Autodesk Inventor part; units mm, degrees
ref_plane "Work Plane1" through (76.2, 0, -20.6375) normal (0, 0, -1) x (-1, 0, 0)
ref_plane "YZ Plane" through (0, 0, 0) normal (1, 0, 0) x (0, 1, 0)
ref_plane "XZ Plane" through (0, 0, 0) normal (0, 1, 0) x (-1, 0, 0)
sketch "Sketch1" plane through (0, 0, 0) normal (0, 1, 0) x (-1, 0, 0)
  line L0 (0, 0) -> (-76.2, 0)
  line L1 (-76.2, 0) -> (-76.2, -41.275)
  line L2 (-76.2, -41.275) -> (0, -41.275)
  line L3 (0, -41.275) -> (0, 0)
  line L4 (0, -39.6875) -> (-76.2, -39.6875)
  line L5 (0, -20.6375) -> (-76.2, -20.6375) construction
  dimension "d0" = 76.2
  dimension "d1" = 41.275
  dimension "d4" = 1.5875
extrude "Extrusion1" add sketch "Sketch1" against normal blind 1.5875
ref_plane "Work Plane1" through (76.2, 0, -20.6375) normal (0, 0, -1) x (-1, 0, 0)
extrude "Extrusion2" add sketch "Sketch1" along normal blind 4.1688 contours L3 L2 L1 L4
sketch "Sketch2" plane through (0, -1.5875, 0) normal (-1, 0, 0) x (0, 0, 1)
  line L0 (-41.275, 5.7563) -> (-39.6875, 5.7563) construction
  line L1 (-39.6875, 1.5875) -> (-39.6875, 5.7563) construction
  circle A0 centre (-39.6875, 4.9625) radius 0.7937
  dimension "d7" = 1.5875
extrude "Extrusion3" add sketch "Sketch2" against normal up to surface (76.2 mm away)
fillet "Fillet1" radius 1.5875 1 edges at (38.1, 4.1688, -41.275)
mirror "Mirror1" about plane through (76.2, 0, -20.6375) normal (0, 0, -1) of "Extrusion2", "Extrusion3", "Fillet1"
fillet "Fillet2" radius 1.5875 2 edges at (38.1, -1.5875, -41.275) (38.1, -1.5875, 0)
fillet "Fillet3" radius 0.7937 2 edges at (38.1, 0, -39.6875) (38.1, 0, -1.5875)
properties part number "Duct Cover"
The listing builds one solid part. Answer for the finished solid, in the listing's coordinates (mm). A direction names the side the tool comes from. Coordinates: 2 decimals unless noted, no trailing zeros. Loops run counter-clockwise (first coordinate to the right, second up) from the corner with the lowest first, then second, coordinate; pieces in that order, holes last. Notation, with made-up numbers: (89, -37.75) - (128, -37.75) arc R25 cw to (128, -2.75) - close; hole circle Ø1 at (-0.5, -2.5). An arc over 180 degrees is marked (long way). Write item = value, one per line.
1) Determine the mould class of faces 4 (the face through (39, 2, -1.588)), 5 (the face through (38.63, -1.11, -0.45)), 6 (the face through (76.2, -0.2, -20.7)) for opening direction Z: pulls with the +Z half, pulls with the -Z half, needs draft (parallel to the pull), parting line crosses it, or undercut.
Responses:
face_4 = undercut
face_5 = pulls with the +Z half
face_6 = needs draft
2) Which of the six approach directions +Z, -Z, +X, -X, +Y, -Y give full straight-line access (tool end or side, diameter ignored) to faces 1 (the face through (38, 1, 0)), 2 (the face through (39, 0, -20)), 3 (the face through (37.57, 3.39, -2.38))?
Responses:
face_1 = +Z, +X, -X, +Y, -Y
face_2 = +X, -X, +Y
face_3 = +X, -X
3) Find the intervals of material crossed by line 1 along Z through (x, y) = (33.5, 1.35) (1 decimal); line 2 along Y through (x, z) = (59.5, -20); line 3 along Z through (x, y) = (71.5, -0.15), in increasing order.
Responses:
line_1 = -41.3 to -39.7, -1.6 to 0
line_2 = -1.59 to 0
line_3 = -41.27 to -0.01
4) This flat-tipped pin is pushed along its axis until it touches: P1, Ø1, axis at y = 2, z = -26, coming from the +X side. Where does it stop, or does it pass through?
Responses:
P1 = through
5) Section B-B (z = -38) is taken. Determine the outline of the cut face in (x, y).
Responses:
outline = (0, -1.59) - (76.2, -1.59) - (76.2, 0) - (0, 0) - close
